For this review, use the dimensioned drawing (mm, ordinates from the lowest corner) and the shaded views. Coordinates: 2 decimals unless noted, no trailing zeros. Write each loop counter-clockwise with the first axis right and the second up, starting at its lowest first coordinate (ties: lowest second). Pieces come first, ordered by that corner, then holes.
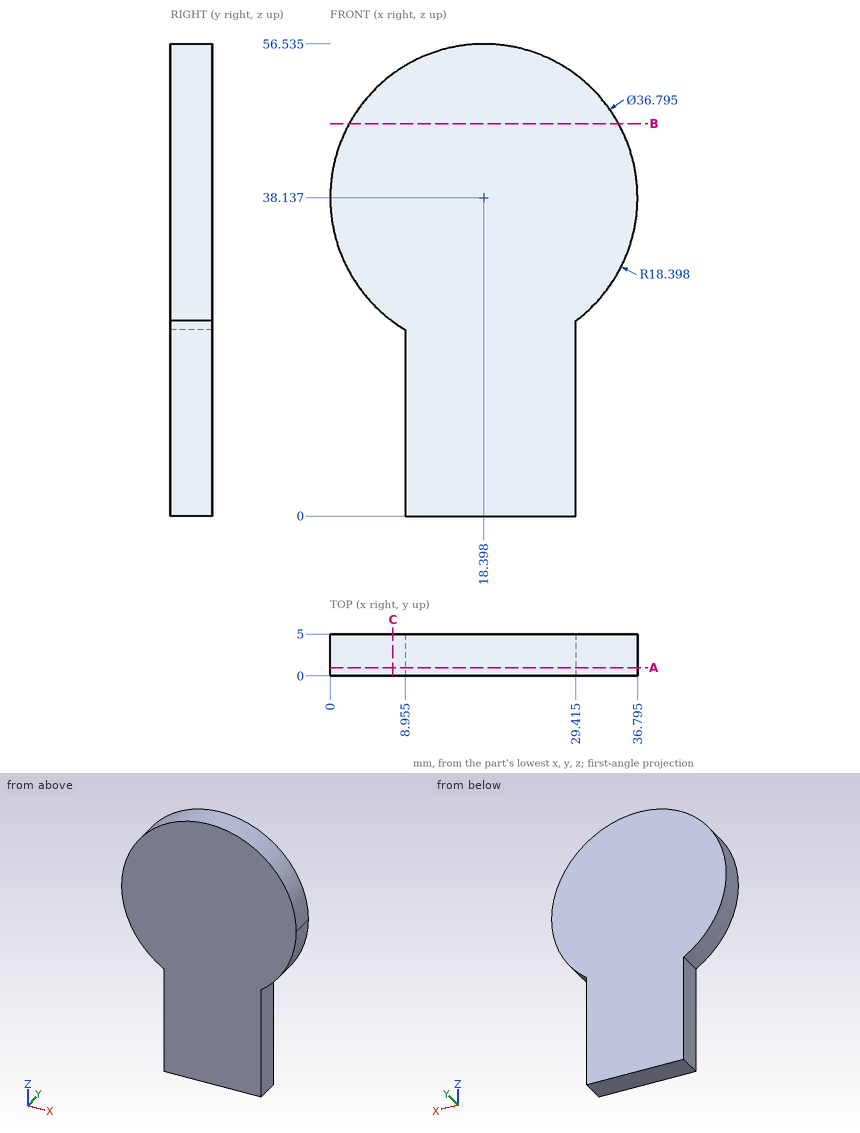
(1) Wall thickness on line 1 (X direction, y = 0.35, z = 37.5) (1 decimal); line 2 (X direction, y = 3.3, z = 16.5) (1 decimal); line 3 (Z direction, x = 12, y = 0.4): over which ranges is each line inside the solid? List them lowest first.
(2) Consider section B-B (z = 47). Give the boundary of the cut face in (x, y) (1 decimal), plus the area to 3 significant figures.
(3) Consider section A-A (y = 1). Give the boundary of the cut face in (x, z) (1 decimal), plus the area to 3 significant figures.
(4) Consider section C-C (x = 7.5). Give the boundary of the cut face in (y, z) (1 decimal), plus the area to 3 significant figures.
(5) Insertion check: pin 1 Ø3 at (y, z) = (4, 29) entering from +X (1 decimal); pin 2 Ø1.5 at (y, z) = (2, 11) entering from -X (1 decimal). Each pin has a flat end and moves straight along its axis. Give the tip position at first contact, or say it passes through.
Results:
1. line 1: x = 0 to 36.8
1. line 2: x = 9 to 29.4
1. line 3: z = 0 to 55.39
2. outline: (2.3, 0) - (34.5, 0) - (34.5, 5) - (2.3, 5) - close
2. area: 161 mm2
3. outline: (9, 0) - (29.4, 0) - (29.4, 23.4) arc R18.4 ccw to (36.8, 38.1) arc R18.4 ccw (long way) to (9, 22.3) - close
3. area: 1,490 mm2
4. outline: (0, 23.3) - (5, 23.3) - (5, 53) - (0, 53) - close
4. area: 148 mm2
5. pin 1: stops at x = 35.1
5. pin 2: stops at x = 9
